Autodesk Inventor part; units mm, degrees
ref_plane "Work Plane1" through (482.6, 0, 0) normal (-1, 0, 0) x (0, 0, 1)
ref_plane "Work Plane2" through (330.2, -584.2, 0) normal (0, -1, 0) x (1, 0, 0)
ref_plane "YZ Plane" through (0, 0, 0) normal (1, 0, 0) x (0, 1, 0)
sketch "Sketch1" plane through (0, 0, 0) normal (0, 0, 1) x (1, 0, 0)
  line L0 (0, 0) -> (965.2, 0)
  line L1 (965.2, 0) -> (965.2, -1168.4)
  line L2 (965.2, -1168.4) -> (0, -1168.4)
  line L3 (0, -1168.4) -> (0, 0)
  dimension "d0" = 965.2
  dimension "d1" = 1168.4
extrude "Extrusion1" add sketch "Sketch1" along normal blind 25.4
sketch "Sketch2" plane through (0, -1168.4, 0) normal (0, -1, 0) x (1, 0, 0)
  line L0 (965.2, 25.4) -> (0, 25.4)
  line L1 (0, 0) -> (965.2, 0)
  line L2 (177.8, 25.4) -> (330.2, 25.4)
  line L3 (330.2, 25.4) -> (330.2, 0)
  line L4 (330.2, 0) -> (177.8, 0)
  line L5 (177.8, 0) -> (177.8, 25.4)
  line L6 (177.8, 12.7) -> (330.2, 12.7)
  line L7 (635, 25.4) -> (787.4, 25.4)
  line L8 (787.4, 25.4) -> (787.4, 0)
  line L9 (787.4, 0) -> (635, 0)
  line L10 (635, 0) -> (635, 25.4)
  line L11 (635, 12.7) -> (787.4, 12.7)
  line L12 (787.4, 12.7) -> (965.2, 12.7)
  line L13 (965.2, 0) -> (965.2, 25.4)
  line L14 (965.2, 0) -> (0, 0)
  line L15 (965.2, 0) -> (965.2, 25.4)
  line L16 (0, 25.4) -> (965.2, 25.4)
  line L17 (0, 0) -> (0, 25.4)
  line L18 (177.8, 12.7) -> (0, 12.7)
  line L19 (0, 0) -> (0, 25.4)
  dimension "d4" = 152.4
  dimension "d5" = 177.8
extrude "Extrusion2" add sketch "Sketch2" along normal blind 50.8 contours L8 L11 L10 L0 | L8 L1 L10 L11 | L3 L6 L5 L0 | L3 L1 L5 L6
sketch "Sketch3" plane through (0, -1168.4, 0) normal (-1, 0, 0) x (0, 0, 1)
  line L0 (0, 0) -> (0, 1168.4)
  line L1 (0, 0) -> (25.4, 0)
  line L2 (25.4, 1168.4) -> (25.4, 0)
  line L3 (0, 1168.4) -> (25.4, 1168.4)
  line L4 (25.4, 1168.4) -> (25.4, 0)
  line L5 (0, 203.2) -> (25.4, 203.2)
  line L6 (25.4, 203.2) -> (25.4, 406.4)
  line L7 (25.4, 406.4) -> (0, 406.4)
  line L8 (0, 406.4) -> (0, 203.2)
  line L9 (0, 0) -> (0, 1168.4)
  line L10 (0, 965.2) -> (25.4, 965.2)
  line L11 (25.4, 965.2) -> (25.4, 762)
  line L12 (25.4, 762) -> (0, 762)
  line L13 (0, 762) -> (0, 965.2)
  dimension "d8" = 203.2
  dimension "d9" = 203.2
  dimension "d12" = 355.6
  dimension "d13" = 203.2
extrude "Extrusion3" cut sketch "Sketch3" against normal blind 25.4 contours L0 L7 L2 L5 | L0 L10 L2 L12
ref_plane "Work Plane1" through (482.6, 0, 0) normal (-1, 0, 0) x (0, 0, 1)
mirror "Mirror1" about plane through (482.6, 0, 0) normal (-1, 0, 0) of "Extrusion3"
ref_plane "Work Plane2" through (330.2, -584.2, 0) normal (0, -1, 0) x (1, 0, 0)
mirror "Mirror2" about plane through (330.2, -584.2, 0) normal (0, -1, 0) of "Extrusion2"
properties part number "rev1 small wall"
Can you work these out from the model? Positions are in its coordinate system, mm. A direction names the side the tool comes from. Round coordinates to 2 decimals unless told otherwise and drop trailing zeros. Order: outer loops, then holes, each group sorted by start corner. A loop starts at its lowest first (then second) coordinate and runs counter-clockwise, first axis right, second up. Notation, with made-up numbers: (-37.5, 60) -> (-16.5, 60) arc R16 cw to (-16.5, 67) -> close; hole circle Ø11 at (8.5, 48). An arc over 180 degrees is marked (long way). Return JSON: item names as keys, results as strings. Group by question number.
1. I need wall thicknesses on line 1 (Y direction, x = 888, z = 2.25); line 2 (X direction, y = -888, z = 5.75). Which ranges of each line are inside material? Lowest first, please. Write a range as [from, to].
2. If we section it at B-B, the plane y = -274.5: Write out the boundary of the cut face in (x, z).
3. We'd pull the mould along Y, two halves only. Please class faces 1 (the face through (710, -1219.2, 13)), 2 (the face through (0, -103, 13)), 3 (the face through (13, -762, 13)): released by +Y, released by -Y, zero draft, split by the parting line, or undercut.
4. Which directions (+Z, -Z, +X, -X, +Y, -Y) give clear straight access to the entire face, cutting with the end or side of a thin tool? Please do faces 4 (the face through (330.2, 25, 13)), 5 (the face through (177.8, 25, 13)), 6 (the face through (953, -203.2, 13)).
5. If we section it at A-A, the plane x = 372.5: Write out the boundary of the cut face in (y, z).
6. Will these pins go through, and if not, where does the flat tip stop? pin 1 (7.5 mm diameter, centred on x = 496.5, z = 18.5, fed in from +Y); pin 2 (3 mm diameter, centred on y = -585.5, z = 9, fed in from -X); pin 3 (7.5 mm diameter, centred on y = -1203, z = 11.5, fed in from -X); pin 4 (7.5 mm diameter, centred on y = -1198.5, z = 6.5, fed in from +X).
Output values:
{
 "1": {"line 1": "[-1168.4, 0]", "line 2": "[25.4, 939.8]"},
 "2": {"outline": "(25.4, 0) -> (939.8, 0) -> (939.8, 25.4) -> (25.4, 25.4) -> close"},
 "3": {"face 1": "released by -Y", "face 2": "zero draft", "face 3": "undercut"},
 "4": {"face 4": "+Z, -Z, +Y", "face 5": "+Z, -Z, -X, +Y", "face 6": "+Z, -Z, +X"},
 "5": {"outline": "(-1168.4, 0) -> (0, 0) -> (0, 25.4) -> (-1168.4, 25.4) -> close"},
 "6": {"pin 1": "y = 0", "pin 2": "x = 0", "pin 3": "x = 177.8", "pin 4": "x = 787.4"}
}
